Read the model definition and answer for the solid it produces. Units are mm, in the model's axes. A direction names the side the tool comes from. Coordinates: 2 decimals unless noted, no trailing zeros. Loops run counter-clockwise (first coordinate to the right, second up) from the corner with the lowest first, then second, coordinate; pieces in that order, holes last. Notation, with made-up numbers: (13, 60.5) - (60, 60.5) arc R32 ccw to (60, 92.5) - close; hole circle Ø11 at (75.25, 43.5). An arc over 180 degrees is marked (long way). Use one line per item in the form item = value.
from build123d import *

# Parameters (mm, degrees)
SKETCH_1_R          = 40
EXTRUDE_1_DEPTH     = 5
EXTRUDE_2_DEPTH     = 20
SKETCH_3_R          = 11
CUT_EXTRUDE_1_DEPTH = 5
EXTRUDE_5_DEPTH     = 5


with BuildPart() as part:
    # 草图1 → 凸台-拉伸1 (new body)
    with BuildSketch(Plane.XY):
        Circle(SKETCH_1_R)
    extrude(amount=EXTRUDE_1_DEPTH)

    # 草图2 → 凸台-拉伸2 (add)
    with BuildSketch(Plane(origin=(0, 0, 0), x_dir=(-1, 0, 0), z_dir=(0, 0, -1))):
        with BuildLine():
            Line((-6.498382723, 17.854159795), (-8.892523726, 24.43200814))
            ThreePointArc((-8.892523726, 24.43200814), (0, 26), (8.892523726, 24.43200814))
            Line((8.892523726, 24.43200814), (6.498382723, 17.854159795))
            ThreePointArc((6.498382723, 17.854159795), (0, 19), (-6.498382723, 17.854159795))
        make_face()
        with BuildLine():
            Line((17.854159795, 6.498382723), (24.43200814, 8.892523726))
            ThreePointArc((24.43200814, 8.892523726), (26, 0), (24.43200814, -8.892523726))
            Line((24.43200814, -8.892523726), (17.854159795, -6.498382723))
            ThreePointArc((17.854159795, -6.498382723), (19, 0), (17.854159795, 6.498382723))
        make_face()
        with BuildLine():
            Line((6.498382723, -17.854159795), (8.892523726, -24.43200814))
            ThreePointArc((8.892523726, -24.43200814), (0, -26), (-8.892523726, -24.43200814))
            Line((-8.892523726, -24.43200814), (-6.498382723, -17.854159795))
            ThreePointArc((-6.498382723, -17.854159795), (0, -19), (6.498382723, -17.854159795))
        make_face()
        with BuildLine():
            Line((-17.854159795, -6.498382723), (-24.43200814, -8.892523726))
            ThreePointArc((-24.43200814, -8.892523726), (-26, 0), (-24.43200814, 8.892523726))
            Line((-24.43200814, 8.892523726), (-17.854159795, 6.498382723))
            ThreePointArc((-17.854159795, 6.498382723), (-19, 0), (-17.854159795, -6.498382723))
        make_face()
    extrude(amount=EXTRUDE_2_DEPTH)

    # 草图3 → 切除-拉伸1 (cut)
    with BuildSketch(Plane(origin=(0, 0, 0), x_dir=(-1, 0, 0), z_dir=(0, 0, -1))):
        Circle(SKETCH_3_R)
    extrude(amount=-CUT_EXTRUDE_1_DEPTH, mode=Mode.SUBTRACT)

    # 草图5 → 凸台-拉伸5 (add)
    with BuildSketch(Plane.XY.offset(5)):
        with BuildLine():
            ThreePointArc((11.876657713, 21.99875), (0, 37.25), (-11.876657713, 21.99875))
            ThreePointArc((-11.876657713, 21.99875), (0, 25), (11.876657713, 21.99875))
        make_face()
        with BuildLine():
            ThreePointArc((21.99875, -11.876657713), (37.25, 0), (21.99875, 11.876657713))
            ThreePointArc((21.99875, 11.876657713), (25, 0), (21.99875, -11.876657713))
        make_face()
        with BuildLine():
            ThreePointArc((-11.876657713, -21.99875), (0, -37.25), (11.876657713, -21.99875))
            ThreePointArc((11.876657713, -21.99875), (0, -25), (-11.876657713, -21.99875))
        make_face()
        with BuildLine():
            ThreePointArc((-21.99875, 11.876657713), (-37.25, 0), (-21.99875, -11.876657713))
            ThreePointArc((-21.99875, -11.876657713), (-25, 0), (-21.99875, 11.876657713))
        make_face()
    extrude(amount=EXTRUDE_5_DEPTH)


solid = part.part
Item 1: The part is cut by section B-B on z = -8. Give the vertices of the cut face in (x, y), plus the area to 3 significant figures.
Results below:
outline = (-24.43, -8.89) - (-17.85, -6.5) arc R19 cw to (-17.85, 6.5) - (-24.43, 8.89) arc R26 ccw to start; (-8.89, -24.43) arc R26 ccw to (8.89, -24.43) - (6.5, -17.85) arc R19 cw to (-6.5, -17.85) - close; (-8.89, 24.43) - (-6.5, 17.85) arc R19 cw to (6.5, 17.85) - (8.89, 24.43) arc R26 ccw to start; (17.85, -6.5) - (24.43, -8.89) arc R26 ccw to (24.43, 8.89) - (17.85, 6.5) arc R19 cw to start
area = 440 mm²
Item 2: Find the intervals of material crossed by L1, parallel to Y at x = 0, z = 2.45; L2, parallel to Z at x = -6, y = 35; L3, parallel to Z at x = -21, y = -21, in increasing order.
Results below:
L1 = -40 to -11, 11 to 40
L2 = 0 to 10
L3 = 0 to 5
Item 3: Which of the six approach directions +Z, -Z, +X, -X, +Y, -Y give full straight-line access (tool end or side, diameter ignored) to faces 4 (the cylindrical face through (-26, 0, -10)), 5 (the flat face through (-21.1, 7.68, -9.86)), 6 (the cylindrical face through (26, 0, -10)), 7 (the cylindrical face through (37.246, -0.312, 7.465)), 8 (the flat face through (21.1, -7.68, -9.86))?
Results below:
face_4 = -Z, -X
face_5 = -Z, +Y
face_6 = -Z, +X
face_7 = +Z
face_8 = -Z, -Y
Item 4: The part is cut by section A-A on x = 0. Give the vertices of the cut face in (y, z), plus the area to 4 significant figures.
Results below:
outline = (-40, 0) - (-26, 0) - (-26, -20) - (-19, -20) - (-19, 0) - (-11, 0) - (-11, 5) - (-25, 5) - (-25, 10) - (-37.25, 10) - (-37.25, 5) - (-40, 5) - close; (11, 0) - (19, 0) - (19, -20) - (26, -20) - (26, 0) - (40, 0) - (40, 5) - (37.25, 5) - (37.25, 10) - (25, 10) - (25, 5) - (11, 5) - close
area = 692.5 mm²
Item 5: For a pull along Y with two mould halves and no side action, classify faces 1 (the flat face through (-21.189, -7.712, -9.86)), 2 (the cylindrical face through (0, -19, -10)), 3 (the cylindrical face through (0, 26, -10)) as +Y half, -Y half, draft (parallel to the pull), parting line (faces both ways), or undercut.
Results below:
face_1 = -Y half
face_2 = undercut
face_3 = +Y half
Item 6: Each of these flat-tipped pins is pushed along its axis until it touches: P1, Ø1.5, axis at x = -7.5, z = -7, coming from the +Y side; P2, Ø5, axis at x = 16.5, z = -12, coming from the +Y side; P3, Ø1, axis at y = 5, z = 4, coming from the +X side. Where does it stop, or does it pass through?
Results below:
P1 = 25.11
P2 = 6.92
P3 = 39.75
Item 7: The part is cut by section D-D on x = -28. Give the vertices of the cut face in (y, z), plus the area to 3 significant figures.
Results below:
outline = (-28.57, 0) - (28.57, 0) - (28.57, 5) - (11.88, 5) - (11.88, 10) - (-11.88, 10) - (-11.88, 5) - (-28.57, 5) - close
area = 404 mm²
